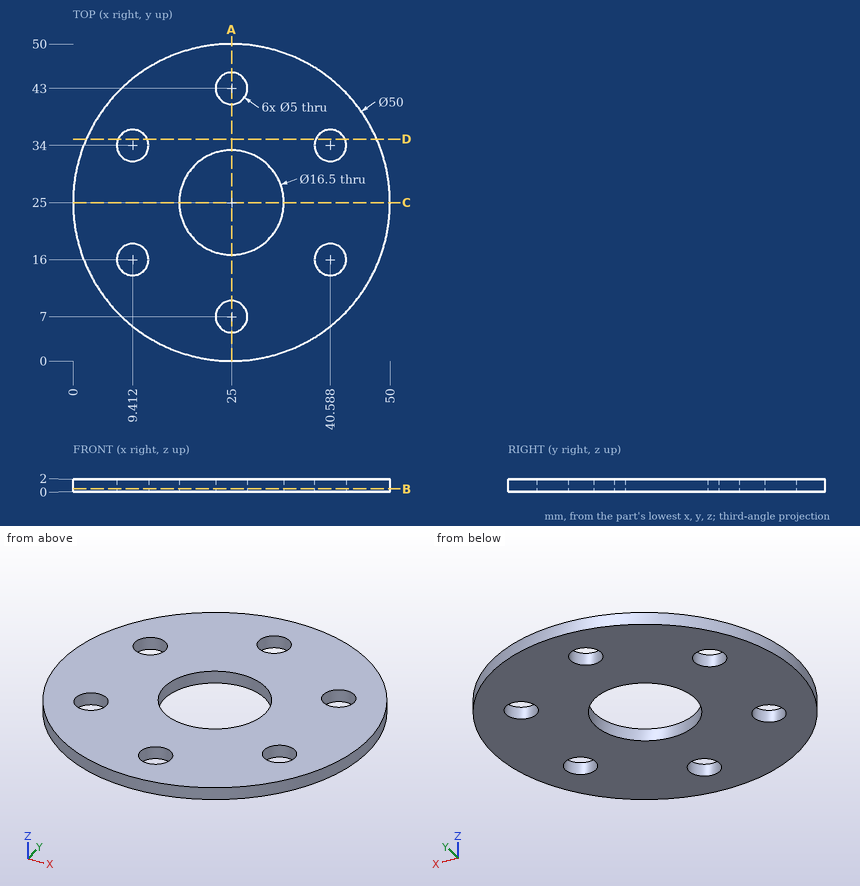
Geometry check sheet. Reference: drawing and pictorial views, mm from the part's lowest x, y, z. Round coordinates to 2 decimals unless told otherwise and drop trailing zeros. Order: outer loops, then holes, each group sorted by start corner. A loop starts at its lowest first (then second) coordinate and runs counter-clockwise, first axis right, second up. Notation, with made-up numbers: M 11.5,21.25 L 16.5,21.25 A32 cw 16.5,50.25 Z; hole C 78,6.25 d1. An arc over 180 degrees is marked long. Answer in a Markdown table with one row per item.
(1) Sectioned sample at A-A, the plane x = 25. Record the cut outline in (y, z).
Responses:
| item | result |
|---|---|
| outline | M 0,0 L 4.5,0 L 4.5,2 L 0,2 Z; M 9.5,0 L 16.75,0 L 16.75,2 L 9.5,2 Z; M 33.25,0 L 40.5,0 L 40.5,2 L 33.25,2 Z; M 45.5,0 L 50,0 L 50,2 L 45.5,2 Z |
(2) Sectioned sample at D-D, the plane y = 35. Record the cut outline in (x, z).
Responses:
| item | result |
|---|---|
| outline | M 2.09,0 L 7.12,0 L 7.12,2 L 2.09,2 Z; M 11.7,0 L 38.3,0 L 38.3,2 L 11.7,2 Z; M 42.88,0 L 47.91,0 L 47.91,2 L 42.88,2 Z |
(3) Go/stop test with flat-tipped pins: P1, Ø6.5, axis at x = 25, y = 7, coming from the -Z side; P2, Ø1, axis at x = 41.5, z = 1.5, coming from the +Y side. Record where each tip stops, or that it passes through.
Responses:
| item | result |
|---|---|
| P1 | stops at z = 0 |
| P2 | stops at y = 44.21 |
(4) Sectioned sample at B-B, the plane z = 0.45. Record the cut outline in (x, y), and give its area (3 significant figures).
Responses:
| item | result |
|---|---|
| outline | C 25,25 d50; hole C 9.41,16 d5; hole C 9.41,34 d5; hole C 25,25 d16.5; hole C 25,7 d5; hole C 25,43 d5; hole C 40.59,16 d5; hole C 40.59,34 d5 |
| area | 1,630 mm² |
(5) Scan lines: probe 1 along Y at (x, z) = (42, 1.65) (1 decimal); probe 2 along Y at (x, z) = (9, 1.65) (1 decimal); probe 3 along X at (y, z) = (34.5, 0.3) (1 decimal). Record each from-to range of solid material in increasing order. Write a range as from..to.
Responses:
| item | result |
|---|---|
| probe 1 | y = 6.7..13.9, 18.1..31.9, 36.1..43.3 |
| probe 2 | y = 5.8..13.5, 18.5..31.5, 36.5..44.2 |
| probe 3 | x = 1.9..7, 11.9..38.1, 43..48.1 |
(6) Sectioned sample at C-C, the plane y = 25. Record the cut outline in (x, z).
Responses:
| item | result |
|---|---|
| outline | M 0,0 L 16.75,0 L 16.75,2 L 0,2 Z; M 33.25,0 L 50,0 L 50,2 L 33.25,2 Z |
